Job drawing, mm, ordinate dimensions from the low corner. One solid piece. Give positions to 0.01 mm unless a question says otherwise; leave off trailing zeros. Order: outer loops, then holes, each group sorted by start corner. A loop starts at its lowest first (then second) coordinate and runs counter-clockwise, first axis right, second up.
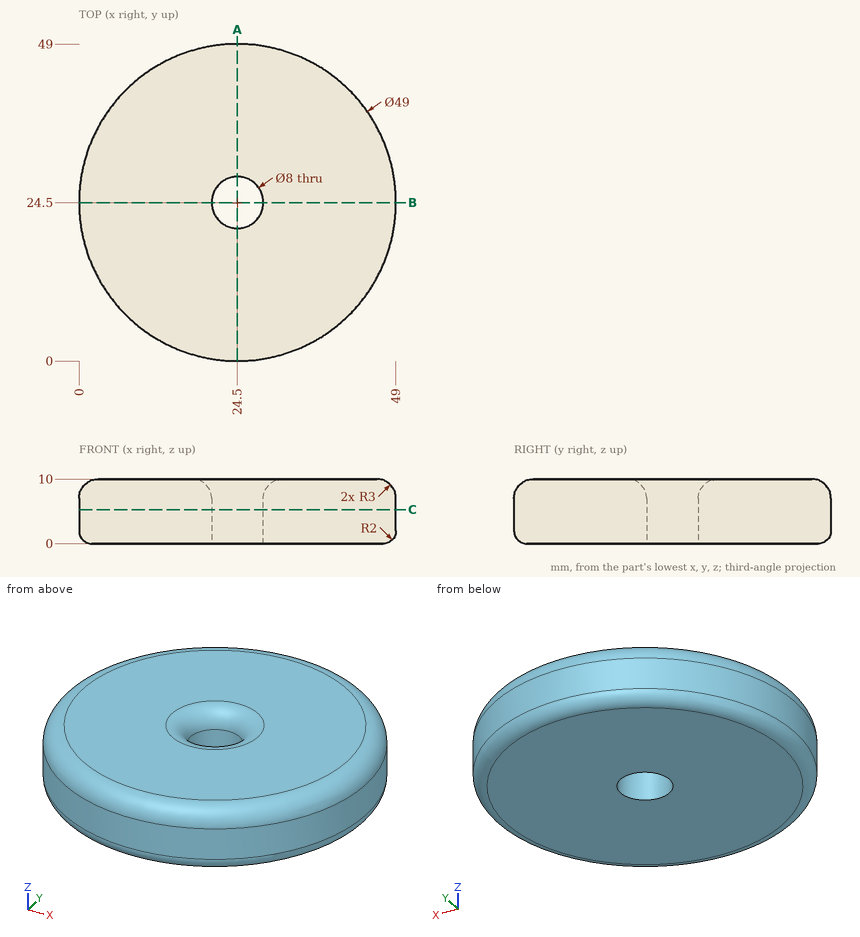
Item 1: Drop flat-ended pins along their axis: P1, Ø4, axis at y = 41, z = 7.5, coming from the -X side; P2, Ø6, axis at y = 9, z = 5, coming from the -X side; P3, Ø4, axis at y = 14, z = 2.5, coming from the +X side; P4, Ø6.5, axis at x = 24.5, y = 24.5, coming from the +Z side. Give the stop position or say it passes through.
Item 2: Band-saw the part on A-A on x = 24.5. List the corners of the cut face in (y, z).
Item 3: Drill centre lines: probe 1 along Y at (x, z) = (24.5, 3.75); probe 2 along X at (y, z) = (22, 1.5); probe 3 along Z at (x, y) = (30, 20.5). Where is each one in solid material? Low to high.
Item 4: Band-saw the part on C-C on z = 5.25. List the corners of the cut face in (x, y).
Working result:
1. P1: stops at x = 4.78
1. P2: stops at x = 3.43
1. P3: stops at x = 47.48
1. P4: passes through
2. outline: (0, 2) arc R2 ccw to (2, 0) - (20.5, 0) - (20.5, 7) arc R3 ccw to (17.5, 10) - (3, 10) arc R3 ccw to (0, 7) - close; (28.5, 0) - (47, 0) arc R2 ccw to (49, 2) - (49, 7) arc R3 ccw to (46, 10) - (31.5, 10) arc R3 ccw to (28.5, 7) - close
3. probe 1: y = 0 to 20.5, 28.5 to 49
3. probe 2: x = 0.19 to 21.38, 27.62 to 48.81
3. probe 3: z = 0 to 9.99
4. outline: circle Ø49 at (24.5, 24.5); hole circle Ø8 at (24.5, 24.5)
